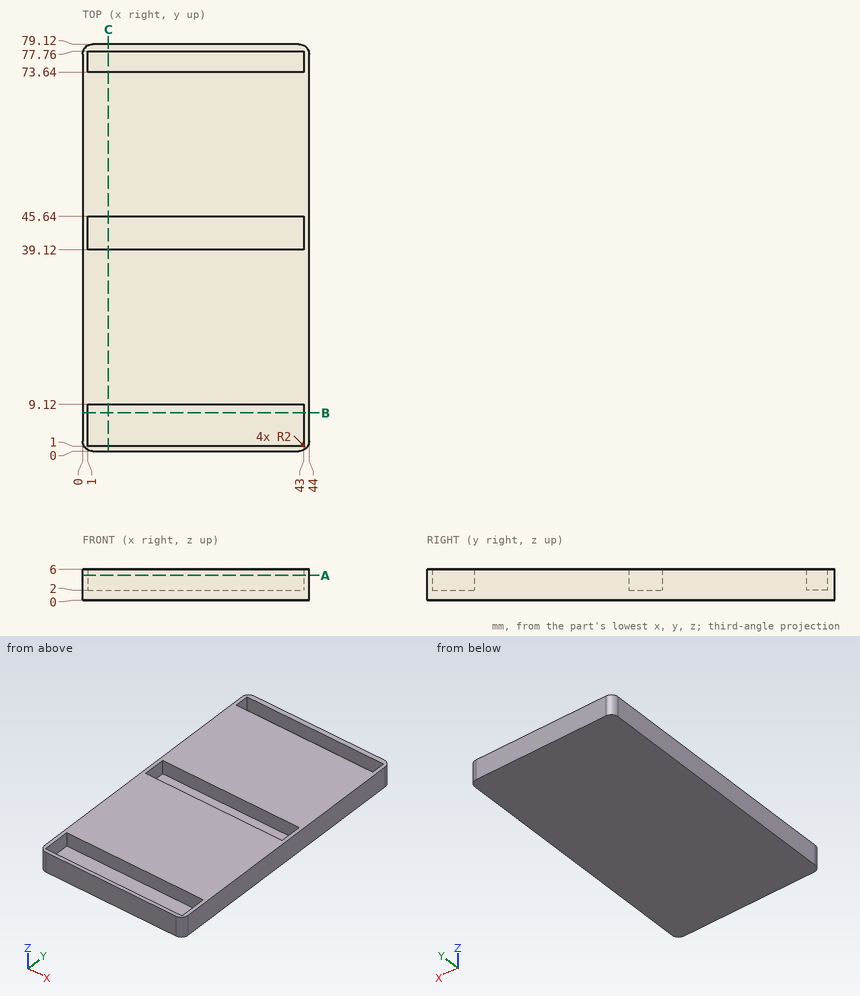
Design review of the part shown in the three views and the two pictorial views. Dimensions are in mm from the part's minimum x, y and z. Round coordinates to 2 decimals unless told otherwise and drop trailing zeros. Loops run counter-clockwise (first coordinate to the right, second up) from the corner with the lowest first, then second, coordinate; pieces in that order, holes last. Notation, with made-up numbers: (45, 74.25) -> (80, 74.25) arc R22 ccw to (80, 111.25) -> close; hole circle Ø5 at (22, 63.25). An arc over 180 degrees is marked (long way). Answer as a JSON object with one key per item and string values. Group by question number.
1) We need section A-A on z = 4.85. Write out the cut boundary in (x, y).
2) We need section C-C on x = 5. Write out the cut boundary in (y, z), then the cut area to 3 significant figures.
3) For pin 1 Ø1.2 at (x, y) = (27, 75.5) entering from +Z, flat-tipped, find the tip position at first contact; note if it passes through.
4) For line 1 (Y direction, x = 9, z = 3.35); line 2 (X direction, y = 39.5, z = 2.6); line 3 (Z direction, x = 8.5, y = 43.5), list the stretches that pass through material, from the lowest coordinate up. Write a range as [from, to].
5) We need section B-B on y = 7.5. Write out the cut boundary in (x, z).
Result set:
{
 "1": {"outline": "(0, 2) arc R2 ccw to (2, 0) -> (42, 0) arc R2 ccw to (44, 2) -> (44, 77.12) arc R2 ccw to (42, 79.12) -> (2, 79.12) arc R2 ccw to (0, 77.12) -> close; hole (1, 1) -> (43, 1) -> (43, 9.12) -> (1, 9.12) -> close; hole (1, 39.12) -> (43, 39.12) -> (43, 45.64) -> (1, 45.64) -> close; hole (1, 73.64) -> (43, 73.64) -> (43, 77.76) -> (1, 77.76) -> close"},
 "2": {"outline": "(0, 0) -> (79.12, 0) -> (79.12, 6) -> (77.76, 6) -> (77.76, 2) -> (73.64, 2) -> (73.64, 6) -> (45.64, 6) -> (45.64, 2) -> (39.12, 2) -> (39.12, 6) -> (9.12, 6) -> (9.12, 2) -> (1, 2) -> (1, 6) -> (0, 6) -> close", "area": "400 mm²"},
 "3": {"pin 1": "z = 2"},
 "4": {"line 1": "[0, 1], [9.12, 39.12], [45.64, 73.64], [77.76, 79.12]", "line 2": "[0, 1], [43, 44]", "line 3": "[0, 2]"},
 "5": {"outline": "(0, 0) -> (44, 0) -> (44, 6) -> (43, 6) -> (43, 2) -> (1, 2) -> (1, 6) -> (0, 6) -> close"}
}
